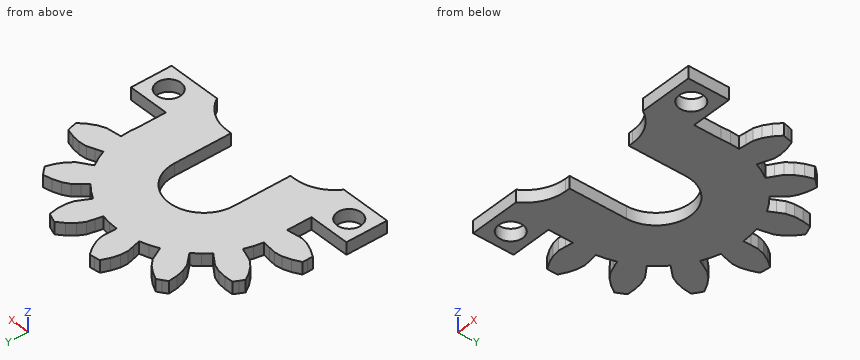
from build123d import *

# Parameters (mm, degrees)
F1_DEPTH  = 1.5
F3_DEPTH  = 1.5
F4_W      = 6.004848
F4_H      = 1.5
F4_W_2    = 6.339723
F5_DEPTH  = 8
F6_W      = 5
F6_H      = 1.5
F7_DEPTH  = 5
F8_R      = 1.5
F9_DEPTH  = 1.5
F10_W     = 5
F10_H     = 5
F10_R     = 1.5
F11_DEPTH = 1.5
F13_DEPTH = 1.5


with BuildPart() as f1:
    # F0 (on Top) → F1 (new body)
    with BuildSketch(Plane.XY):
        Polygon((10.589723, -1.110145), (10.648575, 0), (10.589723, 1.110145), (11.484679, 1.205301), (12.378936, 1.30701), (13.242702, 1.66848), (14.069737, 2.238581), (14.851424, 2.970895), (14.712702, 3.589735), (14.547945, 4.202158), (13.515472, 4.487322), (12.51823, 4.607779), (11.58542, 4.526432), (10.746328, 4.200909), (9.909663, 3.869259), (9.445863, 4.879593), (8.877842, 5.835228), (9.626065, 6.335391), (10.370624, 6.841032), (10.967468, 7.56251), (11.434831, 8.451652), (11.786658, 9.463352), (11.376236, 9.94684), (10.945744, 10.412547), (9.899012, 10.185233), (8.960019, 9.828451), (8.17186, 9.322923), (7.580159, 8.644742), (6.993455, 7.962262), (6.113255, 8.641331), (5.166192, 9.223531), (5.596273, 10.014119), (6.020563, 10.807856), (6.213755, 11.72406), (6.21438, 12.728551), (6.055747, 13.787869), (5.467648, 14.025244), (4.870041, 14.237547), (4.048845, 13.54983), (3.383212, 12.797544), (2.920263, 11.983645), (2.711504, 11.108168), (2.509167, 10.231207), (1.41421, 10.423443), (0.305065, 10.498834), (0.318479, 11.398734), (0.325301, 12.29873), (0.070583, 13.19977), (-0.395674, 14.089492), (-1.028426, 14.953751), (-1.659475, 14.890633), (-2.287292, 14.800897), (-2.694828, 13.810324), (-2.934611, 12.834873), (-2.966295, 11.899058), (-2.744287, 11.026847), (-2.515903, 10.156306), (-3.574776, 9.817671), (-4.591911, 9.36898), (-4.998239, 10.172036), (-5.410447, 10.972114), (-6.054722, 11.651571), (-6.881047, 12.222701), (-7.842962, 12.693909), (-8.372396, 12.344758), (-8.886598, 11.973539), (-8.787111, 10.90704), (-8.546113, 9.931888), (-8.139273, 9.088541), (-7.537358, 8.419408), (-6.930574, 7.754718), (-7.710788, 6.962788), (-8.402899, 6.092806), (-9.135883, 6.615047), (-9.87269, 7.131918), (-10.758927, 7.434137), (-11.756018, 7.555836), (-12.826734, 7.526046), (-13.133265, 6.970848), (-13.416055, 6.403188), (-12.832336, 5.505084), (-12.165768, 4.753627), (-11.413606, 4.195948), (-10.569675, 3.883184), (-9.723497, 3.576617), (-10.046314, 2.512814), (-10.254848, 1.420844), (-11.14657, 1.54263), (-12.039182, 1.657886), (-12.964354, 1.513633), (-13.903791, 1.15802), (-14.838018, 0.634056), (-14.851425, 0), (-14.838018, -0.634056), (-13.903791, -1.15802), (-12.964354, -1.513633), (-12.039182, -1.657886), (-11.14657, -1.54263), (-10.254848, -1.420844), (-10.046314, -2.512814), (-9.723497, -3.576617), (-10.569675, -3.883184), (-11.413606, -4.195948), (-12.165768, -4.753627), (-12.832336, -5.505084), (-13.416055, -6.403188), (-13.133265, -6.970848), (-12.826734, -7.526046), (-11.756018, -7.555836), (-10.758927, -7.434137), (-9.87269, -7.131918), (-9.135883, -6.615047), (-8.402899, -6.092806), (-7.710788, -6.962788), (-6.930574, -7.754718), (-7.537358, -8.419408), (-8.139273, -9.088541), (-8.546113, -9.931888), (-8.787111, -10.90704), (-8.886598, -11.973539), (-8.372396, -12.344758), (-7.842962, -12.693909), (-6.881047, -12.222701), (-6.054722, -11.651571), (-5.410447, -10.972114), (-4.998239, -10.172036), (-4.591911, -9.36898), (-3.574776, -9.817671), (-2.515903, -10.156306), (-2.744287, -11.026847), (-2.966295, -11.899058), (-2.934611, -12.834873), (-2.694828, -13.810324), (-2.287292, -14.800897), (-1.659475, -14.890633), (-1.028426, -14.953751), (-0.395674, -14.089492), (0.070583, -13.19977), (0.325301, -12.29873), (0.318479, -11.398734), (0.305065, -10.498834), (1.41421, -10.423443), (2.509167, -10.231207), (2.711504, -11.108168), (2.920263, -11.983645), (3.383212, -12.797544), (4.048845, -13.54983), (4.870041, -14.237547), (5.467648, -14.025244), (6.055747, -13.787869), (6.21438, -12.728551), (6.213755, -11.72406), (6.020563, -10.807856), (5.596273, -10.014119), (5.166192, -9.223531), (6.113255, -8.641331), (6.993455, -7.962262), (7.580159, -8.644742), (8.17186, -9.322923), (8.960019, -9.828451), (9.899012, -10.185233), (10.945744, -10.412547), (11.376236, -9.94684), (11.786658, -9.463352), (11.434831, -8.451652), (10.967468, -7.56251), (10.370624, -6.841032), (9.626065, -6.335391), (8.877842, -5.835228), (9.445863, -4.879593), (9.909663, -3.869259), (10.746328, -4.200909), (11.58542, -4.526432), (12.51823, -4.607779), (13.515472, -4.487322), (14.547945, -4.202158), (14.712702, -3.589735), (14.851424, -2.970895), (14.069737, -2.238581), (13.242702, -1.66848), (12.378936, -1.30701), (11.484679, -1.205301), align=None)
    extrude(amount=F1_DEPTH)

    # F2 (on face) → F3 (cut, through all)
    with BuildSketch(Plane.XY.offset(1.5)):
        with BuildLine():
            Line((4.25, -1.420844), (4.25, 0))
            ThreePointArc((4.25, 0), (0, 4.25), (-4.25, 0))
            Line((-4.25, 0), (-4.25, -1.420844))
            Line((-4.25, -1.420844), (-10.254848, -1.420844))
            Line((-10.254848, -1.420844), (-10.046314, -2.512814))
            Line((-10.046314, -2.512814), (-9.723497, -3.576617))
            Line((-9.723497, -3.576617), (-10.569675, -3.883184))
            Line((-10.569675, -3.883184), (-11.413606, -4.195948))
            Line((-11.413606, -4.195948), (-12.165768, -4.753627))
            Line((-12.165768, -4.753627), (-12.832336, -5.505084))
            Line((-12.832336, -5.505084), (-13.416055, -6.403188))
            Line((-13.416055, -6.403188), (-13.133265, -6.970848))
            Line((-13.133265, -6.970848), (-12.826734, -7.526046))
            Line((-12.826734, -7.526046), (-11.756018, -7.555836))
            Line((-11.756018, -7.555836), (-10.758927, -7.434137))
            Line((-10.758927, -7.434137), (-9.87269, -7.131918))
            Line((-9.87269, -7.131918), (-9.135883, -6.615047))
            Line((-9.135883, -6.615047), (-8.402899, -6.092806))
            Line((-8.402899, -6.092806), (-7.710788, -6.962788))
            Line((-7.710788, -6.962788), (-6.930574, -7.754718))
            Line((-6.930574, -7.754718), (-7.537358, -8.419408))
            Line((-7.537358, -8.419408), (-8.139273, -9.088541))
            Line((-8.139273, -9.088541), (-8.546113, -9.931888))
            Line((-8.546113, -9.931888), (-8.787111, -10.90704))
            Line((-8.787111, -10.90704), (-8.886598, -11.973539))
            Line((-8.886598, -11.973539), (-8.372396, -12.344758))
            Line((-8.372396, -12.344758), (-7.842962, -12.693909))
            Line((-7.842962, -12.693909), (-6.881047, -12.222701))
            Line((-6.881047, -12.222701), (-6.054722, -11.651571))
            Line((-6.054722, -11.651571), (-5.410447, -10.972114))
            Line((-5.410447, -10.972114), (-4.998239, -10.172036))
            Line((-4.998239, -10.172036), (-4.591911, -9.36898))
            Line((-4.591911, -9.36898), (-3.574776, -9.817671))
            Line((-3.574776, -9.817671), (-2.515903, -10.156306))
            Line((-2.515903, -10.156306), (-2.744287, -11.026847))
            Line((-2.744287, -11.026847), (-2.966295, -11.899058))
            Line((-2.966295, -11.899058), (-2.934611, -12.834873))
            Line((-2.934611, -12.834873), (-2.694828, -13.810324))
            Line((-2.694828, -13.810324), (-2.287292, -14.800897))
            Line((-2.287292, -14.800897), (-1.659475, -14.890633))
            Line((-1.659475, -14.890633), (-1.028426, -14.953751))
            Line((-1.028426, -14.953751), (-0.395674, -14.089492))
            Line((-0.395674, -14.089492), (0.070583, -13.19977))
            Line((0.070583, -13.19977), (0.325301, -12.29873))
            Line((0.325301, -12.29873), (0.318479, -11.398734))
            Line((0.318479, -11.398734), (0.305065, -10.498834))
            Line((0.305065, -10.498834), (1.41421, -10.423443))
            Line((1.41421, -10.423443), (2.509167, -10.231207))
            Line((2.509167, -10.231207), (2.711504, -11.108168))
            Line((2.711504, -11.108168), (2.920263, -11.983645))
            Line((2.920263, -11.983645), (3.383212, -12.797544))
            Line((3.383212, -12.797544), (4.048845, -13.54983))
            Line((4.048845, -13.54983), (4.870041, -14.237547))
            Line((4.870041, -14.237547), (5.467648, -14.025244))
            Line((5.467648, -14.025244), (6.055747, -13.787869))
            Line((6.055747, -13.787869), (6.21438, -12.728551))
            Line((6.21438, -12.728551), (6.213755, -11.72406))
            Line((6.213755, -11.72406), (6.020563, -10.807856))
            Line((6.020563, -10.807856), (5.596273, -10.014119))
            Line((5.596273, -10.014119), (5.166192, -9.223531))
            Line((5.166192, -9.223531), (6.113255, -8.641331))
            Line((6.113255, -8.641331), (6.993455, -7.962262))
            Line((6.993455, -7.962262), (7.580159, -8.644742))
            Line((7.580159, -8.644742), (8.17186, -9.322923))
            Line((8.17186, -9.322923), (8.960019, -9.828451))
            Line((8.960019, -9.828451), (9.899012, -10.185233))
            Line((9.899012, -10.185233), (10.945744, -10.412547))
            Line((10.945744, -10.412547), (11.376236, -9.94684))
            Line((11.376236, -9.94684), (11.786658, -9.463352))
            Line((11.786658, -9.463352), (11.434831, -8.451652))
            Line((11.434831, -8.451652), (10.967468, -7.56251))
            Line((10.967468, -7.56251), (10.370624, -6.841032))
            Line((10.370624, -6.841032), (9.626065, -6.335391))
            Line((9.626065, -6.335391), (8.877842, -5.835228))
            Line((8.877842, -5.835228), (9.445863, -4.879593))
            Line((9.445863, -4.879593), (9.909663, -3.869259))
            Line((9.909663, -3.869259), (10.746328, -4.200909))
            Line((10.746328, -4.200909), (11.58542, -4.526432))
            Line((11.58542, -4.526432), (12.51823, -4.607779))
            Line((12.51823, -4.607779), (13.515472, -4.487322))
            Line((13.515472, -4.487322), (14.547945, -4.202158))
            Line((14.547945, -4.202158), (14.712702, -3.589735))
            Line((14.712702, -3.589735), (14.851424, -2.970895))
            Line((14.851424, -2.970895), (14.069737, -2.238581))
            Line((14.069737, -2.238581), (13.242702, -1.66848))
            Line((13.242702, -1.66848), (12.378936, -1.30701))
            Line((12.378936, -1.30701), (11.484679, -1.205301))
            Line((11.484679, -1.205301), (10.589723, -1.110145))
            Line((10.589723, -1.110145), (10.589723, -1.420844))
            Line((10.589723, -1.420844), (4.25, -1.420844))
        make_face()
    extrude(amount=-F3_DEPTH, mode=Mode.SUBTRACT)

    # F4 (on face) → F5 (join)
    with BuildSketch(Plane.XZ.offset(1.420844)):
        with Locations((-7.252424, 0.75)):
            Rectangle(F4_W, F4_H)
        with Locations((7.4198615, 0.75)):
            Rectangle(F4_W_2, F4_H)
    extrude(amount=F5_DEPTH)

    # F6 (on face) → F7 (join)
    with BuildSketch(Plane.YZ.offset(10.589723)):
        with Locations((-6.920844, 0.75)):
            Rectangle(F6_W, F6_H)
    extrude(amount=F7_DEPTH)

    # F8 (on face) → F9 (cut, through all)
    with BuildSketch(Plane(origin=(0, 0, 0), x_dir=(1, 0, 0), z_dir=(0, 0, -1))):
        with Locations((13.089723, 6.920844)):
            Circle(F8_R)
    extrude(amount=-F9_DEPTH, mode=Mode.SUBTRACT)

    # F10 (on Top) → F11 (join)
    with BuildSketch(Plane.XY):
        with Locations((-12.754848, -6.920844)):
            Rectangle(F10_W, F10_H)
        with Locations((-12.754848, -6.920844)):
            Circle(F10_R, mode=Mode.SUBTRACT)
    extrude(amount=F11_DEPTH)

    # F12 (on face) → F13 (cut, through all)
    with BuildSketch(Plane.XY.offset(1.5)):
        with BuildLine():
            Line((-4.25, -7), (-4.8, -7))
            ThreePointArc((-4.8, -7), (-7.2601036564, -7.6470825875), (-9.0834512169, -9.420844))
            Line((-9.0834512169, -9.420844), (-4.25, -9.420844))
            Line((-4.25, -9.420844), (-4.25, -7))
        make_face()
        with BuildLine():
            Line((4.8, -7), (4.25, -7))
            Line((4.25, -7), (4.25, -9.420844))
            Line((4.25, -9.420844), (9.0834512169, -9.420844))
            ThreePointArc((9.0834512169, -9.420844), (7.2601036564, -7.6470825875), (4.8, -7))
        make_face()
    extrude(amount=-F13_DEPTH, mode=Mode.SUBTRACT)


solid = f1.part
Read the model definition and answer for the solid it produces. Units are mm, in the model's axes. Round coordinates to 2 decimals unless told otherwise and drop trailing zeros. Order: outer loops, then holes, each group sorted by start corner. A loop starts at its lowest first (then second) coordinate and runs counter-clockwise, first axis right, second up. Notation, with made-up numbers: (58, -34) - (95, -34) arc R20 cw to (95, -29) - close; hole circle Ø3 at (55, 70). An arc over 180 degrees is marked (long way). Use one line per item in the form item = value. Start each with the question number.
(1) The part is cut by section C-C (x = 8.5). Give the vertices of the cut face in (y, z).
(2) The part is cut by section B-B (z = 0.45). Count the separate pieces of the cut face and the enclosed holes in it, then the cut area to 3 significant figures.
(3) Find the intervals of material crossed by line 1 along X through (y, z) = (-3, 1); line 2 along X through (y, z) = (10.75, 0.1); line 3 along X through (y, z) = (-4.75, 0.1), in increasing order. Write a range as from..to.
(4) Flat-ended cylindrical pins translate along their axes: pin 1 Ø0.8 at (x, z) = (13, 0.5) entering from +Y; pin 2 Ø0.6 at (x, z) = (-4.5, 0.5) entering from -Y; pin 3 Ø0.8 at (y, z) = (-2.5, 1) entering from +X. Find the tip coordinate at first contact, or state that the pin passes through.
(5) The part is cut by section A-A (y = -6.5). Give the vertices of the cut face in (x, z), then the cut area to 3 significant figures.
Checked values:
q1.outline = (-8.64, 0) - (9.53, 0) - (9.53, 1.5) - (-8.64, 1.5) - close
q2.separate_pieces = 1
q2.enclosed_holes = 2
q2.area = 367 mm^2
q3.line_1 = -10.25..-4.25, 4.25..10.59
q3.line_2 = -8.75..-5.3, -2.67..0.31, 2.63..5.99
q3.line_3 = -15.25..-4.25, 4.25..15.59
q4.pin_1 = 4.6
q4.pin_2 = -7
q4.pin_3 = 10.59
q5.outline = (-15.25, 0) - (-14.19, 0) - (-14.19, 1.5) - (-15.25, 1.5) - close; (-11.32, 0) - (-4.25, 0) - (-4.25, 1.5) - (-11.32, 1.5) - close; (4.25, 0) - (11.65, 0) - (11.65, 1.5) - (4.25, 1.5) - close; (14.53, 0) - (15.59, 0) - (15.59, 1.5) - (14.53, 1.5) - close
q5.area = 24.9 mm^2
